Can you work these out from the drawing? Everything is in mm from the part's minimum corner. Give positions to 0.01 mm unless a question says otherwise; leave off trailing zeros. Write each loop counter-clockwise with the first axis right and the second up, starting at its lowest first coordinate (ties: lowest second). Pieces come first, ordered by that corner, then holes. Notation, with made-up numbers: M -32.5,0 L 22.5,0 A19 cw 22.5,16 Z; hole C 52,-26.5 d8. An arc over 180 degrees is marked long. One line per item, written item: value.
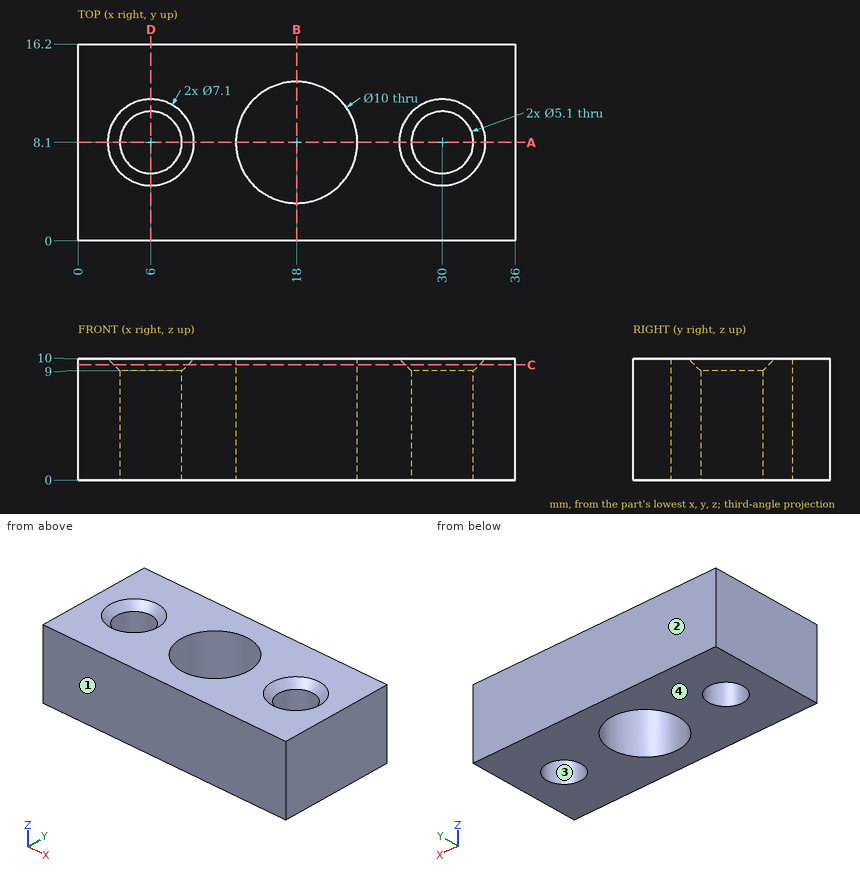
1) If we section it at D-D, the plane x = 6: Write out the boundary of the cut face in (y, z), then the cut area to 3 significant figures.
Outcome:
outline: M 0,0 L 5.55,0 L 5.55,9 L 4.55,10 L 0,10 Z; M 10.65,0 L 16.2,0 L 16.2,10 L 11.65,10 L 10.65,9 Z
area: 110 mm^2
2) If we section it at B-B, the plane x = 18: Write out the boundary of the cut face in (y, z), then the cut area to 3 significant figures.
Outcome:
outline: M 0,0 L 3.1,0 L 3.1,10 L 0,10 Z; M 13.1,0 L 16.2,0 L 16.2,10 L 13.1,10 Z
area: 62.0 mm^2
3) If we section it at C-C, the plane z = 9.5: Write out the boundary of the cut face in (x, y), then the cut area to 3 significant figures.
Outcome:
outline: M 0,0 L 36,0 L 36,16.2 L 0,16.2 Z; hole C 6,8.1 d6.1; hole C 18,8.1 d10; hole C 30,8.1 d6.1
area: 446 mm^2
4) I'm going to push a flat-ended pin straight in: pin 1 (4.5 mm diameter, centred on x = 6, y = 8.1, fed in from -Z). Where does the tip first touch, or does it pass through?
Outcome:
pin 1: passes through
5) We'd pull the mould along Y, two halves only. Please class the marked faces 1, 2, 3 and 4: pulls with the +Y half, pulls with the -Y half, needs draft (parallel to the pull), parting line crosses it, or undercut.
Outcome:
face 1: pulls with the -Y half
face 2: pulls with the +Y half
face 3: undercut
face 4: needs draft
6) Please list where these lines run through material, in increasing order: L1, parallel to X at y = 8, z = 6; L2, parallel to Y at x = 18, z = 3.25; L3, parallel to X at y = 9.25, z = 2. Write a range as from..to.
Outcome:
L1: x = 0..3.45, 8.55..13, 23..27.45, 32.55..36
L2: y = 0..3.1, 13.1..16.2
L3: x = 0..3.72, 8.28..13.13, 22.87..27.72, 32.28..36
7) If we section it at A-A, the plane y = 8.1: Write out the boundary of the cut face in (x, z).
Outcome:
outline: M 0,0 L 3.45,0 L 3.45,9 L 2.45,10 L 0,10 Z; M 8.55,0 L 13,0 L 13,10 L 9.55,10 L 8.55,9 Z; M 23,0 L 27.45,0 L 27.45,9 L 26.45,10 L 23,10 Z; M 32.55,0 L 36,0 L 36,10 L 33.55,10 L 32.55,9 Z
